For this review, take the finished solid that the model builds, in its own axes (mm). Round coordinates to 2 decimals unless told otherwise and drop trailing zeros. Loops run counter-clockwise (first coordinate to the right, second up) from the corner with the lowest first, then second, coordinate; pieces in that order, holes last.
1) Take a section at A-A (z = 221.5). State the section outline as (x, y) points, then the cut area to 3 significant figures.
2) Insertion check: pin 1 (4 mm diameter, centred on x = -49.5, z = 83, fed in from +Y); pin 2 (2 mm diameter, centred on y = 11, z = 200, fed in from -X); pin 3 (12 mm diameter, centred on y = -42, z = 123, fed in from -X). Each pin has a flat end and moves straight along its axis. Give the tip position at first contact, or say it passes through.
3) Wall thickness on L1, parallel to X at y = -25, z = 82; L2, parallel to Y at x = -3, z = 187; L3, parallel to Z at x = -48.5, y = 17.5: over which ranges is each line inside the solid? List them lowest first.
```python
from build123d import *

# Parameters (mm, degrees)
F4_R  = 63.5
F2_R  = 63.5
F0_R  = 63.5
F6_R  = 25.4
F8_R  = 63.5
F10_R = 63.5


with BuildPart() as f5:
    # F4 (on offset) → F5 section 0
    with BuildSketch(Plane.XY.offset(203.2)):
        Circle(F4_R)
    # F2 (on offset) → F5 section 1
    with BuildSketch(Plane.XY.offset(101.6)):
        Circle(F2_R)
    # F0 (on Top) → F5 section 2
    with BuildSketch(Plane.XY):
        Circle(F0_R)
    loft()

    # F6
    f6_edges = [f5.edges().sort_by_distance(p)[0] for p in [
        (-63.5, 0, 0),
    ]]
    fillet(f6_edges, radius=F6_R)

    # F4 (on offset) → F9 section 0
    with BuildSketch(Plane.XY.offset(203.2)):
        Circle(F4_R)
    # F8 (on offset) → F9 section 1
    with BuildSketch(Plane.XY.offset(279.4)):
        Circle(F8_R)
    loft()

    # F10
    f10_edges = [f5.edges().sort_by_distance(p)[0] for p in [
        (-63.5, 0, 279.4),
    ]]
    fillet(f10_edges, radius=F10_R)


solid = f5.part
```
Response:
1. outline: circle Ø126.51 at (0, 0)
1. area: 12,600 mm2
2. pin 1: stops at y = 42.14
2. pin 2: stops at x = -62.71
2. pin 3: stops at x = -52.31
3. L1: x = -58.37 to 58.37
3. L2: y = -63.43 to 63.43
3. L3: z = 3.86 to 252.96
